from build123d import *

# Parameters (mm, degrees)
SKETCH1_W           = 28
SKETCH1_H           = 25
BOSS_EXTRUDE1_DEPTH = 3
FILLET1_R           = 12.5
SKETCH2_W           = 28
SKETCH2_H           = 3
BOSS_EXTRUDE2_DEPTH = 65
SKETCH3_W           = 3
SKETCH3_H           = 48
BOSS_EXTRUDE3_DEPTH = 15.5
SKETCH4_W           = 3
SKETCH4_H           = 48
BOSS_EXTRUDE4_DEPTH = 15.5
SKETCH9_W           = 14.741294127
SKETCH9_H           = 6.665628648
CUT_EXTRUDE1_DEPTH  = 3
SKETCH6_R           = 9
CUT_EXTRUDE2_DEPTH  = 3
CUT_EXTRUDE4_DEPTH  = 3
CUT_EXTRUDE5_DEPTH  = 3
CUT_EXTRUDE8_DEPTH  = 3
FILLET3_R           = 3
FILLET4_R           = 6
FILLET5_R           = 6
FILLET6_R           = 6
FILLET7_R           = 0.5
SKETCH13_R          = 1.5
CUT_EXTRUDE10_DEPTH = 3
SKETCH14_R          = 1
CUT_EXTRUDE11_DEPTH = 3


with BuildPart() as part:
    # Sketch1 → Boss-Extrude1 (new body)
    with BuildSketch(Plane(origin=(0, 0, 0), x_dir=(1, 0, 0), z_dir=(0, 1, 0))):
        Rectangle(SKETCH1_W, SKETCH1_H)
    extrude(amount=BOSS_EXTRUDE1_DEPTH)

    # Fillet1
    fillet1_edges = [part.edges().sort_by_distance(p)[0] for p in [
        (14, 1.5, 12.5),
        (-14, 1.5, 12.5),
    ]]
    fillet(fillet1_edges, radius=FILLET1_R)

    # Sketch2 → Boss-Extrude2 (add)
    with BuildSketch(Plane(origin=(0, 3, 0), x_dir=(1, 0, 0), z_dir=(0, 1, 0))):
        with Locations((0, 11)):
            Rectangle(SKETCH2_W, SKETCH2_H)
    extrude(amount=BOSS_EXTRUDE2_DEPTH)

    # Sketch3 → Boss-Extrude3 (add)
    with BuildSketch(Plane(origin=(14, 0, 0), x_dir=(0, 0, -1), z_dir=(1, 0, 0))):
        with Locations((11, 44)):
            Rectangle(SKETCH3_W, SKETCH3_H)
    extrude(amount=BOSS_EXTRUDE3_DEPTH)

    # Sketch4 → Boss-Extrude4 (add)
    with BuildSketch(Plane.ZY.offset(14)):
        with Locations((-11, 44)):
            Rectangle(SKETCH4_W, SKETCH4_H)
    extrude(amount=BOSS_EXTRUDE4_DEPTH)

    # Sketch9 → Cut-Extrude1 (cut)
    with BuildSketch(Plane.XY.offset(-9.5)):
        with Locations((0.406189009, 49.915136893)):
            Rectangle(SKETCH9_W, SKETCH9_H)
    extrude(amount=-CUT_EXTRUDE1_DEPTH, mode=Mode.SUBTRACT)

    # Sketch6 → Cut-Extrude2 (cut)
    with BuildSketch(Plane.XY.offset(-9.5)):
        with Locations((-13, 50)):
            Circle(SKETCH6_R)
        with Locations((13, 50)):
            Circle(SKETCH6_R)
    extrude(amount=-CUT_EXTRUDE2_DEPTH, mode=Mode.SUBTRACT)

    # Sketch10 → Cut-Extrude4 (cut)
    with BuildSketch(Plane.XY.offset(-9.5)):
        with BuildLine():
            ThreePointArc((4.712414346, 53.509405082), (6.133712339, 55.818427086), (8.178203975, 57.599360703))
            ThreePointArc((8.178203975, 57.599360703), (-3.213e-05, 62.842256013), (-8.178312295, 57.599429431))
            ThreePointArc((-8.178312295, 57.599429431), (-6.134043572, 55.818817949), (-4.71276392, 53.5102305))
            ThreePointArc((-4.71276392, 53.5102305), (-5.8098e-05, 54.842256016), (4.712414346, 53.509405082))
        make_face()
        with BuildLine():
            ThreePointArc((-8.28808236, 42.332025551), (-0.000398085, 36.842256062), (8.286739374, 42.332850969))
            ThreePointArc((8.286739374, 42.332850969), (6.264272315, 44.030915266), (4.821726078, 46.24289531))
            ThreePointArc((4.821726078, 46.24289531), (-5.805e-06, 44.842256013), (-4.821757652, 46.242826582))
            ThreePointArc((-4.821757652, 46.242826582), (-6.264820173, 44.030297102), (-8.28808236, 42.332025551))
        make_face()
        with BuildLine():
            ThreePointArc((-4.821757652, 46.242826582), (-5.805e-06, 44.842256013), (4.821726078, 46.24289531))
            ThreePointArc((4.821726078, 46.24289531), (4.746201964, 46.41185034), (4.674167851, 46.582322569))
            Line((4.674167851, 46.582322569), (-4.674167851, 46.582322569))
            ThreePointArc((-4.674167851, 46.582322569), (-4.746217041, 46.411815659), (-4.821757652, 46.242826582))
        make_face()
        with BuildLine():
            ThreePointArc((4.606501749, 53.247951217), (4.658433625, 53.379093134), (4.712414346, 53.509405082))
            ThreePointArc((4.712414346, 53.509405082), (-5.8098e-05, 54.842256016), (-4.71276392, 53.5102305))
            ThreePointArc((-4.71276392, 53.5102305), (-4.658601912, 53.379508536), (-4.606501749, 53.247951217))
            Line((-4.606501749, 53.247951217), (4.606501749, 53.247951217))
        make_face()
    extrude(amount=-CUT_EXTRUDE4_DEPTH, mode=Mode.SUBTRACT)

    # Sketch11 → Cut-Extrude5 (cut)
    with BuildSketch(Plane.XY.offset(-9.5)):
        Polygon((-29.5, 55.4), (-16.9, 68), (-29.5, 68), align=None)
        Polygon((29.5, 55.4), (29.5, 68), (16.9, 68), align=None)
        Polygon((14, 20), (29.5, 20), (29.5, 35.5), align=None)
        Polygon((-14, 20), (-29.5, 20), (-29.5, 35.5), align=None)
    extrude(amount=-CUT_EXTRUDE5_DEPTH, mode=Mode.SUBTRACT)

    # Sketch12 → Cut-Extrude8 (cut)
    with BuildSketch(Plane.XY.offset(-9.5)):
        with BuildLine():
            Line((-3.25, 33), (-3.25, 23))
            ThreePointArc((-3.25, 23), (-5, 21.25), (-6.75, 23))
            Line((-6.75, 23), (-6.75, 33))
            ThreePointArc((-6.75, 33), (-5, 34.75), (-3.25, 33))
        make_face()
        with BuildLine():
            Line((6.75, 33), (6.75, 23))
            ThreePointArc((6.75, 23), (5, 21.25), (3.25, 23))
            Line((3.25, 23), (3.25, 33))
            ThreePointArc((3.25, 33), (5, 34.75), (6.75, 33))
        make_face()
    extrude(amount=-CUT_EXTRUDE8_DEPTH, mode=Mode.SUBTRACT)

    # Fillet3
    fillet3_edges = [part.edges().sort_by_distance(p)[0] for p in [
        (0, 3, -9.5),
    ]]
    fillet(fillet3_edges, radius=FILLET3_R)

    # Fillet4
    fillet4_edges = [part.edges().sort_by_distance(p)[0] for p in [
        (0, 0, -12.5),
    ]]
    fillet(fillet4_edges, radius=FILLET4_R)

    # Fillet5
    fillet5_edges = [part.edges().sort_by_distance(p)[0] for p in [
        (-14, 20, -11),
        (14, 20, -11),
    ]]
    fillet(fillet5_edges, radius=FILLET5_R)

    # Fillet6
    fillet6_edges = [part.edges().sort_by_distance(p)[0] for p in [
        (-29.5, 55.4, -11),
        (-16.9, 68, -11),
        (29.5, 55.4, -11),
        (16.9, 68, -11),
        (29.5, 35.5, -11),
        (-29.5, 35.5, -11),
    ]]
    fillet(fillet6_edges, radius=FILLET6_R)

    # Fillet7
    fillet7_edges = [part.edges().sort_by_distance(p)[0] for p in [
        (-8.28808236, 42.332025551, -11),
        (8.286739374, 42.332850969, -11),
        (-8.178312295, 57.599429431, -11),
        (8.178203975, 57.599360703, -11),
    ]]
    fillet(fillet7_edges, radius=FILLET7_R)

    # Sketch13 → Cut-Extrude10 (cut)
    with BuildSketch(Plane(origin=(0, 3, 0), x_dir=(1, 0, 0), z_dir=(0, 1, 0))):
        with Locations(Location((0, -1.396515007, 0), (0, 0, 270))):
            Circle(SKETCH13_R)
        with Locations(Location((8.999836974, -1.450685505, 0), (0, 0, 270))):
            Circle(SKETCH13_R)
        with Locations(Location((-8.999405212, -1.499984009, 0), (0, 0, 270))):
            Circle(SKETCH13_R)
    extrude(amount=-CUT_EXTRUDE10_DEPTH, mode=Mode.SUBTRACT)

    # Sketch14 → Cut-Extrude11 (cut)
    with BuildSketch(Plane.XY.offset(-9.5)):
        with Locations((-20.5, 58.25)):
            Circle(SKETCH14_R)
        with Locations((-20.724916228, 41.960213357)):
            Circle(SKETCH14_R)
        with Locations((20.5, 41.75)):
            Circle(SKETCH14_R)
        with Locations((20.715004912, 57.321949454)):
            Circle(SKETCH14_R)
    extrude(amount=-CUT_EXTRUDE11_DEPTH, mode=Mode.SUBTRACT)


solid = part.part
Geometry check sheet. Reference: the model listing, model coordinates, mm. A direction names the side the tool comes from. Round coordinates to 2 decimals unless told otherwise and drop trailing zeros. Order: outer loops, then holes, each group sorted by start corner. A loop starts at its lowest first (then second) coordinate and runs counter-clockwise, first axis right, second up. Notation, with made-up numbers: (19, -17.5) -> (38, -17.5) arc R19 ccw to (38, -7.5) -> close; hole circle Ø2 at (-12, 21.5). An arc over 180 degrees is marked (long way). Use one line per item in the form item = value.
1. Cross-section at A-A, the plane z = 1. Enter the section's corners in (x, y).
Working result:
outline = (-13.96, 0) -> (-10.41, 0) -> (-10.41, 3) -> (-13.96, 3) -> close; (-7.59, 0) -> (-1.45, 0) -> (-1.45, 3) -> (-7.59, 3) -> close; (1.45, 0) -> (7.57, 0) -> (7.57, 3) -> (1.45, 3) -> close; (10.43, 0) -> (13.96, 0) -> (13.96, 3) -> (10.43, 3) -> close
2. Scan lines: line 1 along Y through (x, z) = (-5, -10.5); line 2 along Y through (x, z) = (5, -2); line 3 along Z through (x, y) = (-20.5, 62.5). Record each from-to range of solid material in increasing order. Write a range as from..to.
Working result:
line_1 = 1.53..21.25, 34.75..38.36, 61.33..68
line_2 = 0..3
line_3 = -12.5..-9.5
3. Cross-section at D-D, the plane y = 9. Enter the section's corners in (x, z), plus the area to 3 significant figures.
Working result:
outline = (-14, -12.5) -> (14, -12.5) -> (14, -9.5) -> (-14, -9.5) -> close
area = 84.0 mm^2
4. Mould release check, pull along X, two halves, no side actions. Record for faces 6 (the face through (23.1, 61.8, -11)), 7 (the face through (0.4, 36.6, -12.5)), 8 (the face through (22, 50, -11)), 9 (the face through (4.96, 34.75, -10.98)): pulls with the +X half, pulls with the -X half, needs draft (parallel to the pull), parting line crosses it, or undercut.
Working result:
face_6 = pulls with the +X half
face_7 = needs draft
face_8 = undercut
face_9 = undercut
5. Go/stop test with flat-tipped pins: pin 1 (0.9 mm diameter, centred on y = 27.5, z = -11, fed in from +X); pin 2 (6 mm diameter, centred on y = 18.5, z = -5, fed in from +X); pin 3 (3.5 mm diameter, centred on y = 27.5, z = -11, fed in from -X); pin 4 (2.5 mm diameter, centred on x = 20.72, y = 57.32, fed in from +Z). Record where each tip stops, or that it passes through.
Working result:
pin_1 = 21.95
pin_2 = through
pin_3 = -23.25
pin_4 = -9.5
6. Cross-section at C-C, the plane x = -20.5. Enter the section's corners in (y, z).
Working result:
outline = (26.5, -12.5) -> (40.99, -12.5) -> (40.99, -9.5) -> (26.5, -9.5) -> close; (42.93, -12.5) -> (45.03, -12.5) -> (45.03, -9.5) -> (42.93, -9.5) -> close; (54.97, -12.5) -> (57.25, -12.5) -> (57.25, -9.5) -> (54.97, -9.5) -> close; (59.25, -12.5) -> (64.4, -12.5) -> (64.4, -9.5) -> (59.25, -9.5) -> close
7. Set-up check for faces 1 (the face through (-0.14, 36.843, -10.979)), 2 (the face through (0, 68, -11)), 3 (the face through (-29.5, 46, -11)), 4 (the face through (14, 4.8, -9.5)), 5 (the face through (-14, 4.8, -9.5)): record each of +Z, -Z, +X, -X, +Y, -Y from which the full face is reachable in a straight line by a thin tool's end or side.
Working result:
face_1 = +Z, -Z
face_2 = +Z, -Z, +X, -X, +Y
face_3 = +Z, -Z, -X, +Y, -Y
face_4 = +Z, -Z, +X, -Y
face_5 = +Z, -Z, -X, -Y
8. Cross-section at B-B, the plane x = -13. Enter the section's corners in (y, z), plus the area to 3 significant figures.
Working result:
outline = (0, -6.5) arc R6 ccw to (6, -12.5) -> (41, -12.5) -> (41, -9.5) -> (6, -9.5) arc R3 cw to (3, -6.5) -> (3, 4.9) -> (0, 4.9) -> close; (59, -12.5) -> (68, -12.5) -> (68, -9.5) -> (59, -9.5) -> close
area = 187 mm^2
